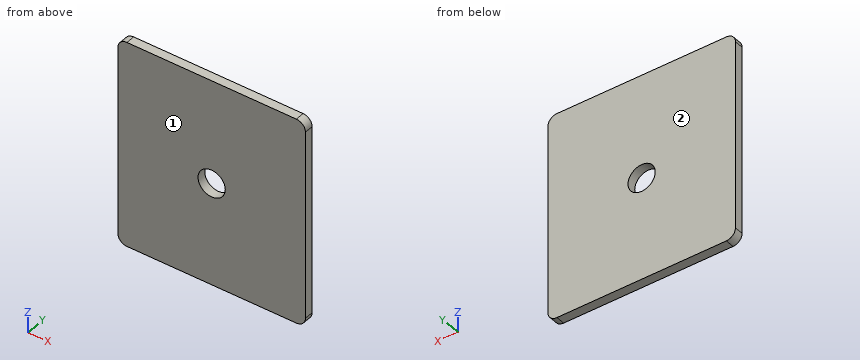
from build123d import *

# Parameters (mm, degrees)
F1_DEPTH = 3
F2_R     = 4.5
F3_DEPTH = 25


with BuildPart() as f1:
    # F0 (on Front) → F1 (new body)
    with BuildSketch(Plane.XZ):
        with BuildLine():
            Line((14.135233, 37.539159), (-41.864767, 37.539159))
            ThreePointArc((-41.864767, 37.539159), (-43.986087, 36.660479), (-44.864767, 34.539159))
            Line((-44.864767, 34.539159), (-44.864767, -27.960841))
            ThreePointArc((-44.864767, -27.960841), (-43.986087, -30.082161), (-41.864767, -30.960841))
            Line((-41.864767, -30.960841), (14.135233, -30.960841))
            ThreePointArc((14.135233, -30.960841), (16.256553, -30.082161), (17.135233, -27.960841))
            Line((17.135233, -27.960841), (17.135233, 34.539159))
            ThreePointArc((17.135233, 34.539159), (16.256553, 36.660479), (14.135233, 37.539159))
        make_face()
    extrude(amount=F1_DEPTH)

    # F2 (on face) → F3 (cut)
    with BuildSketch(Plane.XZ.offset(3)):
        with Locations((-13.864767, 3.039159)):
            Circle(F2_R)
    extrude(amount=-F3_DEPTH, mode=Mode.SUBTRACT)


solid = f1.part
Design review of the part built by this model. Coordinates are the model's own, in mm. Face numbers are marked on the shaded views. Give positions to 0.01 mm unless a question says otherwise; leave off trailing zeros. Order: outer loops, then holes, each group sorted by start corner. A loop starts at its lowest first (then second) coordinate and runs counter-clockwise, first axis right, second up.
1. Add section A-A, the plane x = -13. State the section outline as (y, z) points.
Solution:
outline: (-3, -30.96) - (0, -30.96) - (0, -1.38) - (-3, -1.38) - close; (-3, 7.46) - (0, 7.46) - (0, 37.54) - (-3, 37.54) - close
2. Add section B-B, the plane y = -1.6. State the section outline as (x, z) points, then the cut area to 3 significant figures.
Solution:
outline: (-44.86, -27.96) arc R3 ccw to (-41.86, -30.96) - (14.14, -30.96) arc R3 ccw to (17.14, -27.96) - (17.14, 34.54) arc R3 ccw to (14.14, 37.54) - (-41.86, 37.54) arc R3 ccw to (-44.86, 34.54) - close; hole circle Ø9 at (-13.86, 3.04)
area: 4,180 mm2
3. Mouldability with a two-part tool opening along Y and no side actions: class the marked faces 1 and 2 as +Y half, -Y half, draft (parallel to the pull), parting line (faces both ways), or undercut.
Solution:
face 1: -Y half
face 2: +Y half
4. To check wall thickness, follow L1, parallel to Z at x = -10, y = -1.05; L2, parallel to X at y = -0.8, z = -0.5. State the ranges of each line that lie inside material, in increasing order.
Solution:
L1: z = -30.96 to 0.73, 5.34 to 37.54
L2: x = -44.86 to -16.64, -11.09 to 17.14
